Input: part model. Units: mm. Frame: model coordinates. A direction names the side the tool comes from. Round coordinates to 2 decimals unless told otherwise and drop trailing zeros. Loops run counter-clockwise (first coordinate to the right, second up) from the corner with the lowest first, then second, coordinate; pieces in that order, holes last. Notation, with made-up numbers: (52.25, 19.5) - (71.25, 19.5) arc R27 cw to (71.25, 40.5) - close; hole circle Ø7 at (87, -21.5). An arc over 180 degrees is marked (long way). One line per question, with ' | ' between items. Start each with the question number.
Item 1: First-contact query: pin 1 (12 mm diameter, centred on y = -198, z = -21, fed in from +X); pin 2 (16 mm diameter, centred on x = 59, z = 14.5, fed in from -Y); pin 3 (2 mm diameter, centred on y = -193.5, z = -12.5, fed in from -X). Flat tips, straight axial feed; report the tip coordinate or a pass-through.
Item 2: Set-up query: faces 4 (the face through (-54, -75, 1)), 5 (the face through (0, -33.6, 15)), 6 (the face through (-69.85, -37, 17)), 7 (the face through (54, -75, 1)). Return all of +Z, -Z, +X, -X, +Y, -Y with unobstructed straight access to the full face (end or side cutting, diameter ignored); none if empty.
Item 3: Section A-A, the plane z = 0. Return loops of the section in (x, y) (3 decimals).
Item 4: Section C-C, the plane x = 32.5. Return loops of the section in (y, z), plus the area to 3 significant figures.
Item 5: Draft query along Z for faces 1 (the face through (38, -87, -1)), 2 (the face through (0, -33.6, -15)), 3 (the face through (-1, -49, 36.6)). Return one class per face: pulls with the +Z half, pulls with the -Z half, needs draft (parallel to the pull), parting line crosses it, or undercut.
Item 6: Section B-B, the plane y = -80. Return loops of the section in (x, z).
Item 7: Material intervals for line 1 along Z through (x, y) = (-66, -37); line 2 along X through (y, z) = (-205, 1); line 3 along Z through (x, y) = (0, -120), sorted ascending.
Item 8: Section D-D, the plane y = -37.5. Return loops of the section in (x, z) (3 decimals).
```python
from build123d import *

# Parameters (mm, degrees)
F0_W      = 266.7
F0_H      = 73.2
F1_DEPTH  = 75
F2_W      = 76
F2_H      = 73.2
F3_DEPTH  = 124.6
F4_R      = 58.834667
F5_DEPTH  = 63.5
F6_R      = 62.865407
F7_DEPTH  = 63.5
F3_FACE_W = 76
F3_FACE_H = 73.2
F8_DEPTH  = 25
F9_R      = 76.896223
F9_R_2    = 36.5
F10_DEPTH = 124.5
F11_R     = 27
F12_DEPTH = 191
F13_R     = 7.90944
F14_DEPTH = 291


with BuildPart() as f1:
    # F0 (on Front) → F1 (new body)
    with BuildSketch(Plane.XZ):
        Rectangle(F0_W, F0_H)
    extrude(amount=F1_DEPTH)

    # F2 (on face) → F3 (join)
    with BuildSketch(Plane.XZ.offset(75)):
        Rectangle(F2_W, F2_H)
    extrude(amount=F3_DEPTH)

    # F4 (on face) → F5 (cut)
    with BuildSketch(Plane.YZ.offset(133.35)):
        with Locations((-37.5, 0)):
            Circle(F4_R)
        with BuildLine():
            ThreePointArc((-50.835, 0), (-37.5, 13.335), (-24.165, 0))
            ThreePointArc((-24.165, 0), (-37.5, -13.335), (-50.835, 0))
        make_face(mode=Mode.SUBTRACT)
    extrude(amount=-F5_DEPTH, mode=Mode.SUBTRACT)

    # F6 (on face) → F7 (cut)
    with BuildSketch(Plane(origin=(-133.35, 0, 0), x_dir=(0, -1, 0), z_dir=(-1, 0, 0))):
        with Locations((37.5, 0)):
            Circle(F6_R)
        with BuildLine():
            ThreePointArc((50.835, 0), (37.5, -13.335), (24.165, 0))
            ThreePointArc((24.165, 0), (37.5, 13.335), (50.835, 0))
        make_face(mode=Mode.SUBTRACT)
    extrude(amount=-F7_DEPTH, mode=Mode.SUBTRACT)

    # F3_face (on face) → F8 (join)
    with BuildSketch(Plane.XZ.offset(199.6)):
        Rectangle(F3_FACE_W, F3_FACE_H)
    extrude(amount=F8_DEPTH)

    # F9 (on face) → F10 (cut)
    with BuildSketch(Plane.XZ.offset(224.6)):
        Circle(F9_R)
        Circle(F9_R_2, mode=Mode.SUBTRACT)
    extrude(amount=-F10_DEPTH, mode=Mode.SUBTRACT)

    # F11 (on face) → F12 (cut)
    with BuildSketch(Plane.XZ.offset(224.6)):
        Circle(F11_R)
    extrude(amount=-F12_DEPTH, mode=Mode.SUBTRACT)

    # F13 (on face) → F14 (cut)
    with BuildSketch(Plane.YZ.offset(133.35)):
        with Locations((-37.5, 0)):
            Circle(F13_R)
    extrude(amount=-F14_DEPTH, mode=Mode.SUBTRACT)


solid = f1.part
```
Return value:
1) pin 1: x = 33.28 | pin 2: y = -75 | pin 3: x = -34.64
2) face 4: +Z, -Z, -X, -Y | face 5: -Y | face 6: -X | face 7: +Z, -Z, +X, -Y
3) outline: (-133.35, -50.835) - (-69.85, -50.835) - (-69.85, -75) - (-38, -75) - (-38, -100.1) - (-36.5, -100.1) - (-36.5, -224.6) - (-27, -224.6) - (-27, -45.409) - (-133.35, -45.409) - close; (-133.35, -29.591) - (133.35, -29.591) - (133.35, -24.165) - (69.85, -24.165) - (69.85, 0) - (-69.85, 0) - (-69.85, -24.165) - (-133.35, -24.165) - close; (27, -224.6) - (36.5, -224.6) - (36.5, -100.1) - (38, -100.1) - (38, -75) - (69.85, -75) - (69.85, -50.835) - (133.35, -50.835) - (133.35, -45.409) - (27, -45.409) - close
4) outline: (-224.6, -16.61) - (-100.1, -16.61) - (-100.1, -36.6) - (0, -36.6) - (0, 36.6) - (-100.1, 36.6) - (-100.1, 16.61) - (-224.6, 16.61) - close; hole circle Ø15.82 at (-37.5, 0) | area: 11,300 mm2
5) face 1: needs draft | face 2: undercut | face 3: pulls with the +Z half
6) outline: (-38, -36.6) - (38, -36.6) - (38, 36.6) - (-38, 36.6) - close; hole circle Ø54 at (0, 0)
7) line 1: -36.6 to -7.89, 7.89 to 36.6 | line 2: -36.49 to -26.98, 26.98 to 36.49 | line 3: -36.5 to -27, 27 to 36.5
8) outline: (-133.35, -13.335) - (-69.85, -13.335) - (-69.85, -36.6) - (69.85, -36.6) - (69.85, -13.335) - (133.35, -13.335) - (133.35, -7.909) - (25.816, -7.909) arc R27 cw to (-25.816, -7.909) - (-133.35, -7.909) - close; (-133.35, 7.909) - (-25.816, 7.909) arc R27 cw to (25.816, 7.909) - (133.35, 7.909) - (133.35, 13.335) - (69.85, 13.335) - (69.85, 36.6) - (-69.85, 36.6) - (-69.85, 13.335) - (-133.35, 13.335) - close
